The listing builds one solid part. Answer for the finished solid, in the listing's coordinates (mm). A direction names the side the tool comes from. Coordinates: 2 decimals unless noted, no trailing zeros. Write each loop counter-clockwise with the first axis right and the second up, starting at its lowest first coordinate (ties: lowest second). Pieces come first, ordered by that corner, then holes. Notation, with made-up numbers: M 31.5,64.5 L 63.5,64.5 A22 ccw 63.5,82.5 Z; hole C 32,-22.5 d9. An arc over 180 degrees is marked long. Answer as CSV lines item,"result". Start each with the question number.
```python
from build123d import *

# Parameters (mm, degrees)
F0_W     = 205
F0_H     = 205
F0_W_2   = 195
F0_H_2   = 195
F1_DEPTH = 150
F0_R     = 1.5
F0_W_3   = 49
F0_H_3   = 49
F2_DEPTH = 3


with BuildPart() as f1:
    # F0 (on Top) → F1 (new body)
    with BuildSketch(Plane.XY):
        Rectangle(F0_W, F0_H)
        Rectangle(F0_W_2, F0_H_2, mode=Mode.SUBTRACT)
    extrude(amount=F1_DEPTH)

    # F0 (on Top) → F2 (join)
    with BuildSketch(Plane.XY):
        Rectangle(F0_W_2, F0_H_2)
        with Locations((-95.5, -95.5)):
            Circle(F0_R, mode=Mode.SUBTRACT)
        with Locations((-32.5, -75)):
            Circle(F0_R, mode=Mode.SUBTRACT)
        with Locations((-10, -48.904069)):
            Circle(F0_R, mode=Mode.SUBTRACT)
        with Locations((-48.904069, -10)):
            Circle(F0_R, mode=Mode.SUBTRACT)
        with Locations((32.5, -75)):
            Circle(F0_R, mode=Mode.SUBTRACT)
        with Locations((95.5, -95.5)):
            Circle(F0_R, mode=Mode.SUBTRACT)
        with Locations((10, -48.904069)):
            Circle(F0_R, mode=Mode.SUBTRACT)
        with Locations((48.904069, -10)):
            Circle(F0_R, mode=Mode.SUBTRACT)
        with Locations((-48.904069, 10)):
            Circle(F0_R, mode=Mode.SUBTRACT)
        with Locations((-10, 48.904069)):
            Circle(F0_R, mode=Mode.SUBTRACT)
        with Locations((-95.5, 95.5)):
            Circle(F0_R, mode=Mode.SUBTRACT)
        with Locations((-32.5, 75)):
            Circle(F0_R, mode=Mode.SUBTRACT)
        Rectangle(F0_W_3, F0_H_3, mode=Mode.SUBTRACT)
        with Locations((48.904069, 10)):
            Circle(F0_R, mode=Mode.SUBTRACT)
        with Locations((10, 48.904069)):
            Circle(F0_R, mode=Mode.SUBTRACT)
        with Locations((32.5, 75)):
            Circle(F0_R, mode=Mode.SUBTRACT)
        with Locations((95.5, 95.5)):
            Circle(F0_R, mode=Mode.SUBTRACT)
    extrude(amount=F2_DEPTH)


solid = f1.part
```
1) For a pull along X with two mould halves and no side action, classify faces 1 (the face through (102.5, -1, 74)), 2 (the face through (-1, -97.5, 75)), 3 (the face through (-1, 102.5, 74)) as +X half, -X half, draft (parallel to the pull), parting line (faces both ways), or undercut.
2) The part is cut by section C-C (y = -67). Determine the outline of the cut face in (x, z), then the cut area to 4 significant figures.
3) Find the intervals of material crossed by line 1 (X direction, y = 75, z = 2); line 2 (Y direction, x = 10, z = 2.15); line 3 (Y direction, x = 95.5, z = 0.9), in increasing order. Write a range as from..to.
4) This flat-tipped pin is pushed along its axis until it touches: P1, Ø4, axis at x = -32.5, y = -75, coming from the +Z side. Where does it stop, or does it pass through?
5) The part is cut by section A-A (z = 15). Determine the outline of the cut face in (x, y), then the cut area to 3 significant figures.
6) Which of the six approach directions +Z, -Z, +X, -X, +Y, -Y give full straight-line access (tool end or side, diameter ignored) to faces 4 (the face through (-102.5, -1, 74)), 5 (the face through (97.5, -1, 75))?
7) The part is cut by section B-B (x = -5). Determine the outline of the cut face in (y, z), then the cut area to 3 significant figures.
Completed:
1,face 1,"+X half"
1,face 2,"undercut"
1,face 3,"draft"
2,outline,"M -102.5,0 L 102.5,0 L 102.5,150 L 97.5,150 L 97.5,3 L -97.5,3 L -97.5,150 L -102.5,150 Z"
2,area,"2,085 mm²"
3,line 1,"-102.5..-34, -31..31, 34..102.5"
3,line 2,"-102.5..-50.4, -47.4..-24.5, 24.5..47.4, 50.4..102.5"
3,line 3,"-102.5..-97, -94..94, 97..102.5"
4,P1,"z = 3"
5,outline,"M -102.5,-102.5 L 102.5,-102.5 L 102.5,102.5 L -102.5,102.5 Z; hole M -97.5,-97.5 L 97.5,-97.5 L 97.5,97.5 L -97.5,97.5 Z"
5,area,"4,000 mm²"
6,face 4,"+Z, -Z, -X, +Y, -Y"
6,face 5,"+Z"
7,outline,"M -102.5,0 L -24.5,0 L -24.5,3 L -97.5,3 L -97.5,150 L -102.5,150 Z; M 24.5,0 L 102.5,0 L 102.5,150 L 97.5,150 L 97.5,3 L 24.5,3 Z"
7,area,"1,940 mm²"
